Read the model definition and answer for the solid it produces. Units are mm, in the model's axes. A direction names the side the tool comes from. Coordinates: 2 decimals unless noted, no trailing zeros. Loops run counter-clockwise (first coordinate to the right, second up) from the corner with the lowest first, then second, coordinate; pieces in that order, holes last. Notation, with made-up numbers: (48, 89.5) -> (62, 89.5) arc R29 cw to (62, 128.5) -> close; hole circle Ø6 at (49.5, 23.25). An arc over 180 degrees is marked (long way). Answer as a JSON object with one key per item and string values. Group by question number.
1) Consider probe 1 along X at (y, z) = (-14, -1); probe 2 along Y at (x, z) = (0, -3.25) (3 decimals); probe 3 along X at (y, z) = (25.4, -4.3). Determine where each line is inside the solid, lowest interval first. Write a range as [from, to].
2) Section C-C, the plane y = 25.4 is taken. Give the vertices of the cut face in (x, z).
3) A flat-ended cylindrical pin translates along its axis: P1, Ø2.5, axis at x = -26.8, y = -17.46, coming from the +Z side. Find the tip coordinate at first contact, or state that the pin passes through.
4) Section A-A, the plane x = 0 is taken. Count the separate pieces of the cut face and the enclosed holes in it, plus the area to 3 significant figures.
5) Determine the mould class of faces 1 (the face through (1, -34.925, -3)), 2 (the face through (-1, 34.925, -3)), 3 (the face through (28.086, -17.176, -3.219)) for opening direction Y: released by +Y, released by -Y, zero draft, split by the parting line, or undercut.
6) Section B-B, the plane y = -11.5 is taken. Give the vertices of the cut face in (x, z), plus the area to 3 significant figures.
7) Which of the six approach directions +Z, -Z, +X, -X, +Y, -Y give full straight-line access (tool end or side, diameter ignored) to faces 4 (the face through (-35.56, -19, -3)), 5 (the face through (42.54, 33.114, -3.219))?
Autodesk Inventor part; units mm, degrees
ref_plane "YZ Plane" through (0, 0, 0) normal (1, 0, 0) x (0, 1, 0)
ref_plane "XZ Plane" through (0, 0, 0) normal (0, 1, 0) x (-1, 0, 0)
ref_plane "XY Plane" through (0, 0, 0) normal (0, 0, 1) x (1, 0, 0)
sketch "Sketch1" plane through (0, 0, 0) normal (0, 0, 1) x (1, 0, 0)
  circle A0 centre (0, 0) radius 34.925
  circle A1 centre (0, 0) radius 9.525
  line L0 (-44.45, 34.925) -> (44.45, 34.925)
  line L1 (44.45, 34.925) -> (44.45, -34.925)
  line L2 (44.45, -34.925) -> (-44.45, -34.925)
  line L3 (-44.45, -34.925) -> (-44.45, 34.925)
  line L4 (-40.64, 28.575) -> (-35.56, 28.575)
  line L5 (-35.56, 28.575) -> (-35.56, 9.525)
  line L6 (-35.56, 9.525) -> (-40.64, 9.525)
  line L7 (-40.64, 9.525) -> (-40.64, 28.575)
  arc A2 (-35.56, 28.575) -> (-40.64, 28.575) centre (-38.1, 28.575) ccw
  arc A3 (-40.64, 9.525) -> (-35.56, 9.525) centre (-38.1, 9.525) ccw
  line L8 (35.56, 28.575) -> (40.64, 28.575)
  line L9 (40.64, 28.575) -> (40.64, 9.525)
  line L10 (40.64, 9.525) -> (35.56, 9.525)
  line L11 (35.56, 9.525) -> (35.56, 28.575)
  arc A4 (40.64, 28.575) -> (35.56, 28.575) centre (38.1, 28.575) ccw
  arc A5 (35.56, 9.525) -> (40.64, 9.525) centre (38.1, 9.525) ccw
  line L12 (-40.64, -9.525) -> (-35.56, -9.525)
  line L13 (-35.56, -9.525) -> (-35.56, -28.575)
  line L14 (-35.56, -28.575) -> (-40.64, -28.575)
  line L15 (-40.64, -28.575) -> (-40.64, -9.525)
  arc A6 (-35.56, -9.525) -> (-40.64, -9.525) centre (-38.1, -9.525) ccw
  arc A7 (-40.64, -28.575) -> (-35.56, -28.575) centre (-38.1, -28.575) ccw
  line L16 (35.56, -9.525) -> (40.64, -9.525)
  line L17 (40.64, -9.525) -> (40.64, -28.575)
  line L18 (40.64, -28.575) -> (35.56, -28.575)
  line L19 (35.56, -28.575) -> (35.56, -9.525)
  arc A8 (40.64, -9.525) -> (35.56, -9.525) centre (38.1, -9.525) ccw
  arc A9 (35.56, -28.575) -> (40.64, -28.575) centre (38.1, -28.575) ccw
  point P0 (0, 25.4)
  point P1 (0, -25.4)
  point P2 (-26.797, -17.4625)
  point P3 (-26.797, 17.4625)
  point P4 (26.797, 17.4625)
  point P5 (26.797, -17.4625)
  dimension "d0" = 69.85
  dimension "d1" = 19.05
  dimension "d2" = 25.4
  dimension "d3" = 25.4
  dimension "d4" = 26.797
  dimension "d5" = 17.4625
  dimension "d6" = 17.4625
  dimension "d7" = 26.797
  dimension "d24" = 34.925
  dimension "d25" = 69.85
  dimension "d26" = 44.45
  dimension "d28" = 44.45
  dimension "d30" = 5.08
  dimension "d31" = 19.05
  dimension "d33" = 6.35
  dimension "d34" = 6.35
  dimension "d37" = 76.2
  dimension "d40" = 38.1
extrude "Extrusion1" add sketch "Sketch1" against normal blind 6.35 contours A0
hole "Hole1" at (-26.797, -17.4625, 0) at (-26.797, 17.4625, 0) at (26.797, 17.4625, 0) at (26.797, -17.4625, 0) direction (0, 0, -1) diameter 2.6416 end through all
hole "Hole2" at (0, 25.4, 0) at (0, -25.4, 0) direction (0, 0, -1) diameter 4.826 end through all countersink diameter 9.525 countersink angle 82
extrude "Extrusion2" add sketch "Sketch1" against normal blind 6.35 contours A0 L0 L1 L2 | A0 L2 L3 L0
fillet "Fillet1" radius 6.35 4 edges at (-44.45, 34.925, -3.175) (44.45, 34.925, -3.175) (44.45, -34.925, -3.175) (-44.45, -34.925, -3.175)
properties part number "Dewalt Drill Drive CIMmotor Adaptor rectangle"
Determined:
{
 "1": {"probe 1": "[-44.45, -40.64], [-35.56, 35.56], [40.64, 44.45]", "probe 2": "[-34.925, -27.813], [-22.987, -9.525], [9.525, 22.987], [27.813, 34.925]", "probe 3": "[-44.45, -40.64], [-35.56, -2.41], [2.41, 35.56], [40.64, 44.45]"},
 "2": {"outline": "(-44.45, -6.35) -> (-40.64, -6.35) -> (-40.64, 0) -> (-44.45, 0) -> close; (-35.56, -6.35) -> (-2.41, -6.35) -> (-2.41, -2.7) -> (-4.76, 0) -> (-35.56, 0) -> close; (2.41, -6.35) -> (35.56, -6.35) -> (35.56, 0) -> (4.76, 0) -> (2.41, -2.7) -> close; (40.64, -6.35) -> (44.45, -6.35) -> (44.45, 0) -> (40.64, 0) -> close"},
 "3": {"P1": "through"},
 "4": {"separate pieces": "4", "enclosed holes": "0", "area": "249 mm²"},
 "5": {"face 1": "released by -Y", "face 2": "released by +Y", "face 3": "undercut"},
 "6": {"outline": "(-44.45, -6.35) -> (-40.64, -6.35) -> (-40.64, 0) -> (-44.45, 0) -> close; (-35.56, -6.35) -> (35.56, -6.35) -> (35.56, 0) -> (-35.56, 0) -> close; (40.64, -6.35) -> (44.45, -6.35) -> (44.45, 0) -> (40.64, 0) -> close", "area": "500 mm²"},
 "7": {"face 4": "+Z, -Z", "face 5": "+Z, -Z, +X, +Y"}
}
